Geometry: final body of the model. Coordinates: model frame, mm. A direction names the side the tool comes from. Round coordinates to 2 decimals unless told otherwise and drop trailing zeros. Loops run counter-clockwise (first coordinate to the right, second up) from the corner with the lowest first, then second, coordinate; pieces in that order, holes last. Notation, with made-up numbers: (47, 16.5) -> (95, 16.5) arc R12 cw to (95, 22.5) -> close; hole circle Ø2 at (59, 18). An arc over 180 degrees is marked (long way). Answer in a Markdown table with one row per item.
```python
from build123d import *
from OCP.BRepFilletAPI import BRepFilletAPI_MakeChamfer

# Parameters (mm, degrees)
BOSS_EXTRUDE1_DEPTH = 8
SKETCH3_W           = 17
SKETCH3_H           = 16
CUT_EXTRUDE1_DEPTH  = 8
SKETCH3_5_R         = 1.5
CUT_EXTRUDE3_DEPTH  = 8
SKETCH3_6_R         = 2.75
CUT_EXTRUDE4_DEPTH  = 6
CHAMFER1_SIZE       = 4
CHAMFER1_SIZE2      = 3.356398525
SKETCH4_W           = 18
SKETCH4_H           = 60
CUT_EXTRUDE6_DEPTH  = 6
SKETCH5_W           = 4
SKETCH5_H           = 20.5
CUT_EXTRUDE8_DEPTH  = 8
FILLET1_R           = 2
SKETCH6_W           = 22
SKETCH6_H           = 25
CUT_EXTRUDE10_DEPTH = 2


with BuildPart() as part:
    # Sketch1 → Boss-Extrude1 (new body)
    with BuildSketch(Plane.XY):
        with BuildLine():
            Line((-32, 13.367307057), (-29.257142857, 12.152097325))
            ThreePointArc((-29.257142857, 12.152097325), (-31.914285714, -0.405069911), (-29.257142857, -12.962237146))
            Line((-29.257142857, -12.962237146), (-32, -14.177446879))
            ThreePointArc((-32, -14.177446879), (-0.914285714, -34.405069911), (30.171428571, -14.177446879))
            Line((30.171428571, -14.177446879), (27.428571429, -12.962237146))
            ThreePointArc((27.428571429, -12.962237146), (30.085714286, -0.405069911), (27.428571429, 12.152097325))
            Line((27.428571429, 12.152097325), (30.171428571, 13.367307057))
            ThreePointArc((30.171428571, 13.367307057), (-0.914285714, 33.594930089), (-32, 13.367307057))
        make_face()
    extrude(amount=BOSS_EXTRUDE1_DEPTH)

    # Sketch3 → Cut-Extrude1 (cut)
    with BuildSketch(Plane.XY.offset(8)):
        with Locations((-21.5, -0.405069911)):
            Rectangle(SKETCH3_W, SKETCH3_H)
        with Locations((19.671428571, -0.405069911)):
            Rectangle(SKETCH3_W, SKETCH3_H)
    extrude(amount=-CUT_EXTRUDE1_DEPTH, mode=Mode.SUBTRACT)

    # Sketch3<5> → Cut-Extrude3 (cut)
    with BuildSketch(Plane.XY.offset(8)):
        with Locations(Location((19.085714286, 19.594930089, 0), (0, 0, 180))):
            Circle(SKETCH3_5_R)
        with Locations((-20.914285714, 19.594930089)):
            Circle(SKETCH3_5_R)
        with Locations((19.085714286, -20.405069911)):
            Circle(SKETCH3_5_R)
        with Locations((-20.914285714, -20.405069911)):
            Circle(SKETCH3_5_R)
    extrude(amount=-CUT_EXTRUDE3_DEPTH, mode=Mode.SUBTRACT)

    # Sketch3<6> → Cut-Extrude4 (cut)
    with BuildSketch(Plane.XY.offset(8)):
        with Locations((19.085714286, 19.594930089)):
            Circle(SKETCH3_6_R)
        with Locations((19.085714286, -20.405069911)):
            Circle(SKETCH3_6_R)
        with Locations((-20.914285714, 19.594930089)):
            Circle(SKETCH3_6_R)
        with Locations((-20.914285714, -20.405069911)):
            Circle(SKETCH3_6_R)
    extrude(amount=-CUT_EXTRUDE4_DEPTH, mode=Mode.SUBTRACT)

    # Chamfer1: one chamfer whose edges measure the first distance from different faces: ONE call of the kernel's chamfer builder (chamfer() names one face for all edges)
    chamfer1_edges_1 = [part.edges().sort_by_distance(p)[0] for p in [
        (28.8, 12.759702191, 8),
    ]]
    chamfer1_side_1 = [part.faces().sort_by_distance(p)[0] for p in [
        (28.8, 12.759702191, 4),
    ]]
    chamfer1_edges_2 = [part.edges().sort_by_distance(p)[0] for p in [
        (-30.628571429, 12.759702191, 8),
    ]]
    chamfer1_side_2 = [part.faces().sort_by_distance(p)[0] for p in [
        (-30.628571429, 12.759702191, 4),
    ]]
    chamfer1_edges_3 = [part.edges().sort_by_distance(p)[0] for p in [
        (-30.628571429, -13.569842013, 8),
    ]]
    chamfer1_side_3 = [part.faces().sort_by_distance(p)[0] for p in [
        (-30.628571429, -13.569842013, 4),
    ]]
    chamfer1_edges_4 = [part.edges().sort_by_distance(p)[0] for p in [
        (28.8, -13.569842013, 8),
    ]]
    chamfer1_side_4 = [part.faces().sort_by_distance(p)[0] for p in [
        (28.8, -13.569842013, 4),
    ]]
    chamfer1 = BRepFilletAPI_MakeChamfer(part.part.solid().wrapped)
    for e in chamfer1_edges_1:
        chamfer1.Add(CHAMFER1_SIZE, CHAMFER1_SIZE2, e.wrapped, chamfer1_side_1[0].wrapped)  # the first distance lies on this face
    for e in chamfer1_edges_2:
        chamfer1.Add(CHAMFER1_SIZE, CHAMFER1_SIZE2, e.wrapped, chamfer1_side_2[0].wrapped)  # the first distance lies on this face
    for e in chamfer1_edges_3:
        chamfer1.Add(CHAMFER1_SIZE, CHAMFER1_SIZE2, e.wrapped, chamfer1_side_3[0].wrapped)  # the first distance lies on this face
    for e in chamfer1_edges_4:
        chamfer1.Add(CHAMFER1_SIZE, CHAMFER1_SIZE2, e.wrapped, chamfer1_side_4[0].wrapped)  # the first distance lies on this face
    add(Compound.cast(chamfer1.Shape()), mode=Mode.REPLACE)

    # Sketch4 → Cut-Extrude6 (cut)
    with BuildSketch(Plane.XY):
        with Locations((-0.914285714, -0.405069911)):
            Rectangle(SKETCH4_W, SKETCH4_H)
    extrude(amount=CUT_EXTRUDE6_DEPTH, mode=Mode.SUBTRACT)

    # Sketch5 → Cut-Extrude8 (cut)
    with BuildSketch(Plane.XY):
        with Locations((2.085714286, -0.405069911)):
            Rectangle(SKETCH5_W, SKETCH5_H)
        with Locations((-3.914285714, -0.405069911)):
            Rectangle(SKETCH5_W, SKETCH5_H)
    extrude(amount=CUT_EXTRUDE8_DEPTH, mode=Mode.SUBTRACT)

    # Fillet1
    fillet1_edges = [part.edges().sort_by_distance(p)[0] for p in [
        (0.085714286, -10.655069911, 7),
        (4.085714286, -10.655069911, 7),
        (4.085714286, 9.844930089, 7),
        (0.085714286, 9.844930089, 7),
        (-1.914285714, -10.655069911, 7),
        (-5.914285714, -10.655069911, 7),
        (-1.914285714, 9.844930089, 7),
        (-5.914285714, 9.844930089, 7),
    ]]
    fillet(fillet1_edges, radius=FILLET1_R - 0.0001)  # a hair under: the kernel refuses the full size

    # Sketch6 → Cut-Extrude10 (cut)
    with BuildSketch(Plane(origin=(0, 0, 0), x_dir=(-1, 0, 0), z_dir=(0, 0, -1))):
        with Locations((0.914285714, -0.405069911)):
            Rectangle(SKETCH6_W, SKETCH6_H)
    extrude(amount=-CUT_EXTRUDE10_DEPTH, mode=Mode.SUBTRACT)


solid = part.part
```
Item 1: Pin query (flat end, axial travel): pin 1 Ø1.6 at (y, z) = (-4.5, 1.5) entering from +X; pin 2 Ø2 at (x, z) = (-23.5, 3.5) entering from -Y; pin 3 Ø3 at (y, z) = (-23, 2) entering from +X. Return the tip coordinate at first contact, or that it passes through.
Answer:
| item | result |
|---|---|
| pin 1 | stops at x = 29.91 |
| pin 2 | stops at y = -26.67 |
| pin 3 | stops at x = 25.75 |
Item 2: Cut plane C-C (z = 0.75). Count the separate pieces of the cut face and the enclosed holes in it, then the cut area to 3 significant figures.
Answer:
| item | result |
|---|---|
| separate pieces | 1 |
| enclosed holes | 7 |
| area | 1,720 mm² |
Item 3: Draft query along X for faces 1 (the face through (-5.914, -1, 7)), 2 (the face through (-22, -8.405, 4)), 3 (the face through (-0.37, 33.59, 3.94)), 4 (the face through (12, 8, 0)). Return one class per face: pulls with the +X half, pulls with the -X half, needs draft (parallel to the pull), parting line crosses it, or undercut.
Answer:
| item | result |
|---|---|
| face 1 | undercut |
| face 2 | undercut |
| face 3 | parting line crosses it |
| face 4 | needs draft |
Item 4: Cut plane D-D (y = 11). Output: boundary loops of the cut face in (x, z).
Answer:
| item | result |
|---|---|
| outline | (-29.74, 0) -> (-11.91, 0) -> (-11.91, 2) -> (-9.91, 2) -> (-9.91, 6) -> (8.09, 6) -> (8.09, 2) -> (10.09, 2) -> (10.09, 0) -> (27.91, 0) -> (27.91, 8) -> (-29.74, 8) -> close |
Item 5: Line query: probe 1 along X at (y, z) = (19, 4); probe 2 along Y at (x, z) = (-20, 5.5); probe 3 along X at (y, z) = (-22.5, 7.25). Output: solid intervals per line, ascending. Write a range as [from, to].
Answer:
| item | result |
|---|---|
| probe 1 | x = [-28.83, -23.6], [-18.23, -9.91], [8.09, 16.4], [21.77, 27] |
| probe 2 | y = [-28.54, -23], [-17.81, -8.41], [7.59, 17], [22.19, 27.73] |
| probe 3 | x = [-26.76, -22.7], [-19.13, 17.3], [20.87, 24.93] |
Item 6: Reachability of faces 5 (the face through (-2.516, -10.085, 7.014)), 6 (the face through (-1, 0, 6)), 7 (the face through (-20, -22, 2)) from +Z, -Z, +X, -X, +Y, -Y: full face, straight path, thin tool, end or side. Return the list, or none.
Answer:
| item | result |
|---|---|
| face 5 | +Z, -Z |
| face 6 | -Z |
| face 7 | +Z |
Item 7: Cut plane A-A (x = -24.5). Output: boundary loops of the cut face in (y, z).
Answer:
| item | result |
|---|---|
| outline | (-24.89, 0) -> (-8.41, 0) -> (-8.41, 8) -> (-24.89, 8) -> close; (7.59, 0) -> (24.08, 0) -> (24.08, 8) -> (7.59, 8) -> close |
Item 8: Cut plane B-B (y = 1.5). Output: boundary loops of the cut face in (x, z), then the cut area to 3 significant figures.
Answer:
| item | result |
|---|---|
| outline | (-31.86, 0) -> (-30, 0) -> (-30, 8) -> (-31.86, 8) -> close; (-13, 0) -> (-11.91, 0) -> (-11.91, 2) -> (-9.91, 2) -> (-9.91, 6) -> (-5.91, 6) -> (-5.91, 8) -> (-13, 8) -> close; (-1.91, 6) -> (0.09, 6) -> (0.09, 8) -> (-1.91, 8) -> close; (4.09, 6) -> (8.09, 6) -> (8.09, 2) -> (10.09, 2) -> (10.09, 0) -> (11.17, 0) -> (11.17, 8) -> (4.09, 8) -> close; (28.17, 0) -> (30.03, 0) -> (30.03, 8) -> (28.17, 8) -> close |
| area | 91.1 mm² |
